Job drawing, mm, ordinate dimensions from the low corner. One solid piece. Give positions to 0.01 mm unless a question says otherwise; leave off trailing zeros. Order: outer loops, then holes, each group sorted by start corner. A loop starts at its lowest first (then second) coordinate and runs counter-clockwise, first axis right, second up. Notation, with made-up numbers: M 53,73 L 57,73 A21 cw 57,80 Z; hole C -30.75,-9 d11. An arc over 180 degrees is marked long. One line per question, with ' | ' between items.
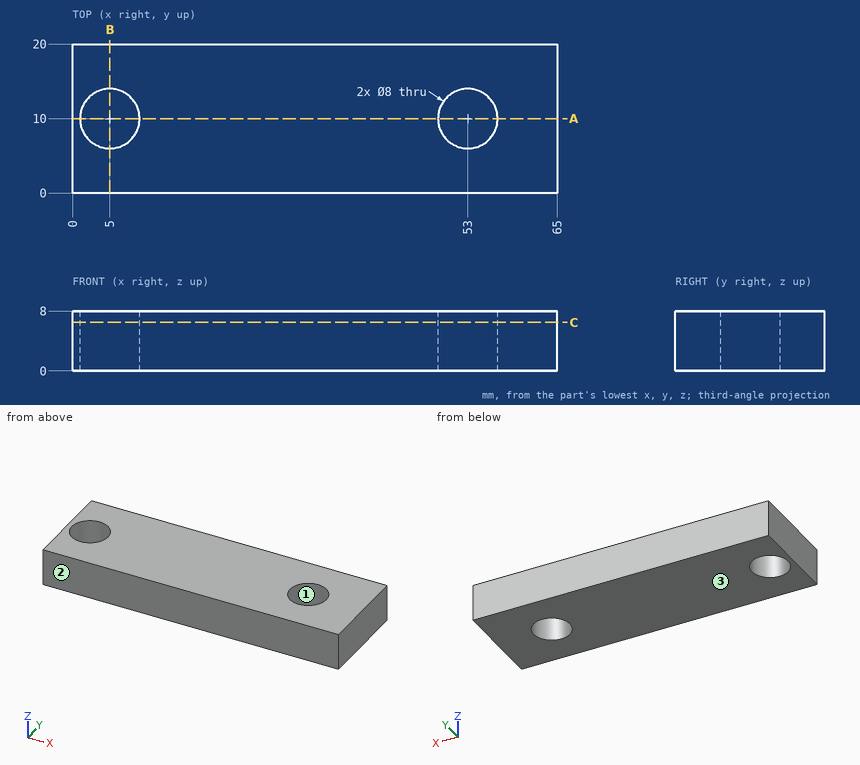
1. Probe L1, parallel to X at y = 9.75, z = 5; L2, parallel to X at y = 8.25, z = 6.5; L3, parallel to Y at x = 53, z = 2.25. List the from-to ranges inside material, lowest first. Write a range as from..to.
Worked out:
L1: x = 0..1.01, 8.99..49.01, 56.99..65 | L2: x = 0..1.4, 8.6..49.4, 56.6..65 | L3: y = 0..6, 14..20
2. Slice it at A-A on y = 10. Give the cut face in (x, z), then the cut area to 3 significant figures.
Worked out:
outline: M 0,0 L 1,0 L 1,8 L 0,8 Z; M 9,0 L 49,0 L 49,8 L 9,8 Z; M 57,0 L 65,0 L 65,8 L 57,8 Z | area: 392 mm2
3. Slice it at C-C on z = 6.5. Give the cut face in (x, y).
Worked out:
outline: M 0,0 L 65,0 L 65,20 L 0,20 Z; hole C 5,10 d8; hole C 53,10 d8
4. Slice it at B-B on x = 5. Give the cut face in (y, z), then the cut area to 3 significant figures.
Worked out:
outline: M 0,0 L 6,0 L 6,8 L 0,8 Z; M 14,0 L 20,0 L 20,8 L 14,8 Z | area: 96.0 mm2
5. Mould opens along Y. For the marked faces 1, 2 and 3 say: released by +Y, released by -Y, zero draft, split by the parting line, or undercut.
Worked out:
face 1: undercut | face 2: released by -Y | face 3: zero draft
